For this review, take the finished solid that the model builds, in its own axes (mm). A direction names the side the tool comes from. Coordinates: 2 decimals unless noted, no trailing zeros. Order: outer loops, then holes, each group sorted by start corner. A loop starts at its lowest first (then second) coordinate and runs counter-clockwise, first axis right, second up.
from build123d import *

# Parameters (mm, degrees)
F3_DEPTH = 7
F4_R     = 1
F5_DEPTH = 25


with BuildPart() as f1:
    # F0 (on Top) → F1 (revolve)
    with BuildSketch(Plane.XY):
        Polygon((-45.818276, -33.398176), (-45.818276, -22.798176), (-50.818276, -22.798176), (-50.818276, -32.798176), (-53.318276, -32.798176), (-53.318276, -34.298176), (-49.318276, -34.298176), (-48.359134, -33.398176), align=None)
    revolve(axis=Axis((-45.818276, -28.098176, 0), (0, -1, 0)))

    # F2 (on face) → F3 (cut)
    with BuildSketch(Plane(origin=(0, -22.798176, 0), x_dir=(-1, 0, 0), z_dir=(0, 1, 0))):
        with BuildLine():
            Line((43.568276, 1.984313), (43.568276, -1.984313))
            ThreePointArc((43.568276, -1.984313), (45.818276, -3), (48.068276, -1.984313))
            Line((48.068276, -1.984313), (48.068276, 1.984313))
            ThreePointArc((48.068276, 1.984313), (45.818276, 3), (43.568276, 1.984313))
        make_face()
    extrude(amount=-F3_DEPTH, mode=Mode.SUBTRACT)

    # F4 (on face) → F5 (cut)
    with BuildSketch(Plane.XZ.offset(33.398176)):
        with Locations((-45.818276, 0)):
            Circle(F4_R)
    extrude(amount=-F5_DEPTH, mode=Mode.SUBTRACT)


solid = f1.part
1. Take a section at D-D, the plane z = 4. Give the boundary of the cut face in (x, y).
Answer below:
outline: (-52.16, -34.3) - (-39.47, -34.3) - (-39.47, -32.8) - (-42.82, -32.8) - (-42.82, -22.8) - (-48.82, -22.8) - (-48.82, -32.8) - (-52.16, -32.8) - close
2. Machinability: for faces 1 (the face through (-48.1, -22.798, 2.2)), 2 (the face through (-43.568, -26, 0)), 3 (the face through (-47, -33.398, 0)), which of the approach directions +Z, -Z, +X, -X, +Y, -Y give a long, thin tool a straight path to every point of the face, cutting with its end or side? Answer none if there is none.
Answer below:
face 1: +Z, -Z, +X, -X, +Y
face 2: +Y
face 3: -Y
3. Take a section at C-C, the plane x = -50.5. Give the boundary of the cut face in (y, z), plus the area to 3 significant figures.
Answer below:
outline: (-34.3, -5.86) - (-32.8, -5.86) - (-32.8, -1.76) - (-22.8, -1.76) - (-22.8, 1.76) - (-32.8, 1.76) - (-32.8, 5.86) - (-34.3, 5.86) - close
area: 52.7 mm2
4. The part is to be moulded in two halves that separate along X. For faces 4 (the face through (-38.326, -33.559, -0.33)), 5 (the face through (-49, -34.298, 2)), 6 (the face through (-45.8, -26.2, -3)), say which applies: +X half, -X half, draft (parallel to the pull), parting line (faces both ways), or undercut.
Answer below:
face 4: parting line
face 5: draft
face 6: undercut
5. Take a section at A-A, the plane z = 0. Give the boundary of the cut face in (x, y).
Answer below:
outline: (-53.32, -34.3) - (-49.32, -34.3) - (-48.36, -33.4) - (-46.82, -33.4) - (-46.82, -29.8) - (-48.07, -29.8) - (-48.07, -22.8) - (-50.82, -22.8) - (-50.82, -32.8) - (-53.32, -32.8) - close; (-44.82, -33.4) - (-43.28, -33.4) - (-42.32, -34.3) - (-38.32, -34.3) - (-38.32, -32.8) - (-40.82, -32.8) - (-40.82, -22.8) - (-43.57, -22.8) - (-43.57, -29.8) - (-44.82, -29.8) - close
6. Take a section at B-B, the plane y = -32. Give the boundary of the cut face in (x, z).
Answer below:
outline: circle Ø10 at (-45.82, 0); hole circle Ø2 at (-45.82, 0)
7. Clearance check with flat-ended pins moving along their axes: pin 1 Ø2.5 at (x, z) = (-45.5, 1) entering from -Y; pin 2 Ø3 at (y, z) = (-25.5, 0.5) entering from -X; pin 3 Ø6 at (y, z) = (-29, 0) entering from +X. State where each tip first meets the part, or that it passes through.
Answer below:
pin 1: stops at y = -33.4
pin 2: stops at x = -50.82
pin 3: stops at x = -40.82
8. To check wall thickness, follow L1, parallel to Z at x = -45.75, y = -24; L2, parallel to Y at x = -41.5, z = 5.5; L3, parallel to Z at x = -44.5, y = -26. State the ranges of each line that lie inside material, in increasing order.
Answer below:
L1: z = -5 to -3, 3 to 5
L2: y = -34.3 to -32.8
L3: z = -4.82 to -2.69, 2.69 to 4.82
